Here's how the part is built. I have some questions about the finished solid (model axes, mm). Face numbers are marked on the shaded views. A direction names the side the tool comes from. Round coordinates to 2 decimals unless told otherwise and drop trailing zeros. Write each loop counter-clockwise with the first axis right and the second up, starting at its lowest first coordinate (ties: lowest second). Pieces come first, ordered by that corner, then holes. Notation, with made-up numbers: (4, 86) -> (31, 86) arc R15 cw to (31, 101) -> close; hole circle Ø10 at (83, 46). An arc over 180 degrees is marked (long way). Put each result on its own line as item: value. Start each with the question number.
1) Will these pins go through, and if not, where does the flat tip stop? P1, Ø8, axis at x = -17.5, z = 22.5, coming from the -Y side; P2, Ø8, axis at x = 16.5, z = 18, coming from the -Y side.
2) Which directions (+Z, -Z, +X, -X, +Y, -Y) give clear straight access to the entire face, cutting with the end or side of a thin tool? Please do the marked faces 1 and 2.
3) If I drill on line 1 along X through (y, z) = (-12, 22.5); line 2 along Z through (x, y) = (13.5, -4.25); line 3 along Z through (x, y) = (-27, -5.75), over which ranges is the centre line in solid material (lowest first)? Write a range as [from, to].
4) I want a section at C-C, the plane y = -9.5. List the corners of the cut face in (x, z) for me, then the cut area to 3 significant figures.
5) I want a section at B-B, the plane z = -9. List the corners of the cut face in (x, y) for me, then the cut area to 3 significant figures.
6) I want a section at A-A, the plane x = 4. List the corners of the cut face in (y, z) for me, then the cut area to 3 significant figures.
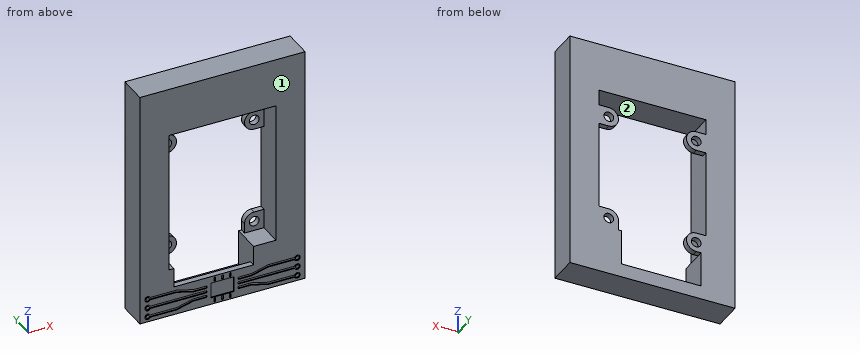
from build123d import *

# Parameters (mm, degrees)
F0_W     = 85
F0_H     = 123
F1_DEPTH = 15
F0_R     = 2.5
F2_DEPTH = 3
F3_START = 12
F0_W_2   = 41
F0_H_2   = 8
F3_DEPTH = 3
F4_R     = 0.875
F5_DEPTH = 0.5


with BuildPart() as f1:
    # F0 (on Front) → F1 (new body)
    with BuildSketch(Plane.XZ):
        with Locations((-6.7032766342, -3.7414353937)):
            Rectangle(F0_W, F0_H)
        Polygon((-34.2032766342, 24.7585646063), (-34.2032766342, 32.7585646063), (20.7967233658, 32.7585646063), (20.7967233658, 24.7585646063), (20.7967233658, 14.7585646063), (20.7967233658, -30.2414353937), (20.7967233658, -40.2414353937), (15.7967233658, -40.2414353937), (10.7967233658, -40.2414353937), (9.2967233658, -40.2414353937), (9.2967233658, -50.2414353937), (9.2967233658, -58.2414353937), (-31.7032766342, -58.2414353937), (-31.7032766342, -50.2414353937), (-31.7032766342, -40.2414353937), (-34.2032766342, -40.2414353937), (-34.2032766342, -30.2414353937), (-34.2032766342, 14.7585646063), align=None, mode=Mode.SUBTRACT)
    extrude(amount=F1_DEPTH)

    # F0 (on Front) → F2 (join)
    with BuildSketch(Plane.XZ):
        with BuildLine():
            Line((-29.2032766342, 24.7585646063), (-34.2032766342, 24.7585646063))
            Line((-34.2032766342, 24.7585646063), (-34.2032766342, 14.7585646063))
            Line((-34.2032766342, 14.7585646063), (-29.2032766342, 14.7585646063))
            ThreePointArc((-29.2032766342, 14.7585646063), (-24.2032766342, 19.7585646063), (-29.2032766342, 24.7585646063))
        make_face()
        with Locations((-29.2032766342, 19.7585646063)):
            Circle(F0_R, mode=Mode.SUBTRACT)
        with BuildLine():
            Line((20.7967233658, 14.7585646063), (20.7967233658, 24.7585646063))
            Line((20.7967233658, 24.7585646063), (15.7967233658, 24.7585646063))
            ThreePointArc((15.7967233658, 24.7585646063), (10.7967233658, 19.7585646063), (15.7967233658, 14.7585646063))
            Line((15.7967233658, 14.7585646063), (20.7967233658, 14.7585646063))
        make_face()
        with Locations((15.7967233658, 19.7585646063)):
            Circle(F0_R, mode=Mode.SUBTRACT)
        with BuildLine():
            Line((20.7967233658, -40.2414353937), (20.7967233658, -30.2414353937))
            Line((20.7967233658, -30.2414353937), (15.7967233658, -30.2414353937))
            ThreePointArc((15.7967233658, -30.2414353937), (12.2611894599, -31.7059014878), (10.7967233658, -35.2414353937))
            Line((10.7967233658, -35.2414353937), (10.7967233658, -40.2414353937))
            Line((10.7967233658, -40.2414353937), (15.7967233658, -40.2414353937))
            Line((15.7967233658, -40.2414353937), (20.7967233658, -40.2414353937))
        make_face()
        with Locations((15.7967233658, -35.2414353937)):
            Circle(F0_R, mode=Mode.SUBTRACT)
        with BuildLine():
            Line((-29.2032766342, -30.2414353937), (-34.2032766342, -30.2414353937))
            Line((-34.2032766342, -30.2414353937), (-34.2032766342, -40.2414353937))
            Line((-34.2032766342, -40.2414353937), (-31.7032766342, -40.2414353937))
            Line((-31.7032766342, -40.2414353937), (-29.2032766342, -40.2414353937))
            ThreePointArc((-29.2032766342, -40.2414353937), (-24.2032766342, -35.2414353937), (-29.2032766342, -30.2414353937))
        make_face()
        with Locations((-29.2032766342, -35.2414353937)):
            Circle(F0_R, mode=Mode.SUBTRACT)
    extrude(amount=F2_DEPTH)

    # F0 (on Front) → F3 (join)
    with BuildSketch(Plane.XZ.offset(F3_START)):
        with Locations((-11.2032766342, -54.2414353937)):
            Rectangle(F0_W_2, F0_H_2)
    extrude(amount=F3_DEPTH)

    # F4 (on face) → F5 (cut)
    with BuildSketch(Plane.XZ.offset(15)):
        with BuildLine():
            Line((-30.2032766342, -52.3664353937), (-43.8396876199, -52.3664353937))
            ThreePointArc((-43.8396876199, -52.3664353937), (-46.7032766342, -52.9914353937), (-43.8396876199, -53.6164353937))
            Line((-43.8396876199, -53.6164353937), (-30.2032766342, -53.6164353937))
            Line((-30.2032766342, -53.6164353937), (-21.7032766342, -55.8664353937))
            Line((-21.7032766342, -55.8664353937), (-15.2032766342, -55.8664353937))
            ThreePointArc((-15.2032766342, -55.8664353937), (-14.5782766342, -55.2414353937), (-15.2032766342, -54.6164353937))
            Line((-15.2032766342, -54.6164353937), (-21.7032766342, -54.6164353937))
            Line((-21.7032766342, -54.6164353937), (-30.2032766342, -52.3664353937))
        make_face()
        with Locations((-45.2032766342, -52.9914353937)):
            Circle(F4_R, mode=Mode.SUBTRACT)
        with BuildLine():
            Line((-15.2032766342, -57.1164353937), (-43.8396876199, -57.1164353937))
            ThreePointArc((-43.8396876199, -57.1164353937), (-46.7032766342, -57.7414353937), (-43.8396876199, -58.3664353937))
            Line((-43.8396876199, -58.3664353937), (-15.2032766342, -58.3664353937))
            ThreePointArc((-15.2032766342, -58.3664353937), (-14.5782766342, -57.7414353937), (-15.2032766342, -57.1164353937))
        make_face()
        with Locations((-45.2032766342, -57.7414353937)):
            Circle(F4_R, mode=Mode.SUBTRACT)
        with BuildLine():
            Line((-30.2032766342, -61.8664353937), (-43.8396876199, -61.8664353937))
            ThreePointArc((-43.8396876199, -61.8664353937), (-46.7032766342, -62.4914353937), (-43.8396876199, -63.1164353937))
            Line((-43.8396876199, -63.1164353937), (-30.2032766342, -63.1164353937))
            Line((-30.2032766342, -63.1164353937), (-21.7032766342, -60.8664353937))
            Line((-21.7032766342, -60.8664353937), (-15.2032766342, -60.8664353937))
            ThreePointArc((-15.2032766342, -60.8664353937), (-14.5782766342, -60.2414353937), (-15.2032766342, -59.6164353937))
            Line((-15.2032766342, -59.6164353937), (-21.7032766342, -59.6164353937))
            Line((-21.7032766342, -59.6164353937), (-30.2032766342, -61.8664353937))
        make_face()
        with Locations((-45.2032766342, -62.4914353937)):
            Circle(F4_R, mode=Mode.SUBTRACT)
        with BuildLine():
            Line((16.7967233658, -53.6164353937), (30.4331343515, -53.6164353937))
            ThreePointArc((30.4331343515, -53.6164353937), (33.2967233658, -52.9914353937), (30.4331343515, -52.3664353937))
            Line((30.4331343515, -52.3664353937), (16.7967233658, -52.3664353937))
            Line((16.7967233658, -52.3664353937), (8.2967233658, -54.6164353937))
            Line((8.2967233658, -54.6164353937), (1.7967233658, -54.6164353937))
            ThreePointArc((1.7967233658, -54.6164353937), (1.1717233658, -55.2414353937), (1.7967233658, -55.8664353937))
            Line((1.7967233658, -55.8664353937), (8.2967233658, -55.8664353937))
            Line((8.2967233658, -55.8664353937), (16.7967233658, -53.6164353937))
        make_face()
        with Locations((31.7967233658, -52.9914353937)):
            Circle(F4_R, mode=Mode.SUBTRACT)
        with BuildLine():
            Line((1.7967233658, -58.3664353937), (30.4331343515, -58.3664353937))
            ThreePointArc((30.4331343515, -58.3664353937), (33.2967233658, -57.7414353937), (30.4331343515, -57.1164353937))
            Line((30.4331343515, -57.1164353937), (1.7967233658, -57.1164353937))
            ThreePointArc((1.7967233658, -57.1164353937), (1.1717233658, -57.7414353937), (1.7967233658, -58.3664353937))
        make_face()
        with Locations((31.7967233658, -57.7414353937)):
            Circle(F4_R, mode=Mode.SUBTRACT)
        with BuildLine():
            Line((16.7967233658, -63.1164353937), (30.4331343515, -63.1164353937))
            ThreePointArc((30.4331343515, -63.1164353937), (33.2967233658, -62.4914353937), (30.4331343515, -61.8664353937))
            Line((30.4331343515, -61.8664353937), (16.7967233658, -61.8664353937))
            Line((16.7967233658, -61.8664353937), (8.2967233658, -59.6164353937))
            Line((8.2967233658, -59.6164353937), (1.7967233658, -59.6164353937))
            ThreePointArc((1.7967233658, -59.6164353937), (1.1717233658, -60.2414353937), (1.7967233658, -60.8664353937))
            Line((1.7967233658, -60.8664353937), (8.2967233658, -60.8664353937))
            Line((8.2967233658, -60.8664353937), (16.7967233658, -63.1164353937))
        make_face()
        with Locations((31.7967233658, -62.4914353937)):
            Circle(F4_R, mode=Mode.SUBTRACT)
        Polygon((-12.7032766342, -61.7414353937), (-6.7032766342, -61.7414353937), (-0.7032766342, -61.7414353937), (-0.7032766342, -57.7414353937), (-0.7032766342, -53.7414353937), (-6.7032766342, -53.7414353937), (-12.7032766342, -53.7414353937), (-12.7032766342, -57.7414353937), align=None)
        with BuildLine():
            Line((-6.2032766342, -52.7414353937), (-6.2032766342, -51.4914353937))
            ThreePointArc((-6.2032766342, -51.4914353937), (-6.7032766342, -50.9914353937), (-7.2032766342, -51.4914353937))
            Line((-7.2032766342, -51.4914353937), (-7.2032766342, -52.7414353937))
            ThreePointArc((-7.2032766342, -52.7414353937), (-6.7032766342, -53.2414353937), (-6.2032766342, -52.7414353937))
        make_face()
        with BuildLine():
            Line((-2.2032766342, -52.7414353937), (-2.2032766342, -51.4914353937))
            ThreePointArc((-2.2032766342, -51.4914353937), (-2.7032766342, -50.9914353937), (-3.2032766342, -51.4914353937))
            Line((-3.2032766342, -51.4914353937), (-3.2032766342, -52.7414353937))
            ThreePointArc((-3.2032766342, -52.7414353937), (-2.7032766342, -53.2414353937), (-2.2032766342, -52.7414353937))
        make_face()
        with BuildLine():
            ThreePointArc((-11.2032766342, -52.7414353937), (-10.7032766342, -53.2414353937), (-10.2032766342, -52.7414353937))
            Line((-10.2032766342, -52.7414353937), (-10.2032766342, -51.4914353937))
            ThreePointArc((-10.2032766342, -51.4914353937), (-10.7032766342, -50.9914353937), (-11.2032766342, -51.4914353937))
            Line((-11.2032766342, -51.4914353937), (-11.2032766342, -52.7414353937))
        make_face()
        with BuildLine():
            Line((-11.2032766342, -62.7414353937), (-11.2032766342, -63.9914353937))
            ThreePointArc((-11.2032766342, -63.9914353937), (-10.7032766342, -64.4914353937), (-10.2032766342, -63.9914353937))
            Line((-10.2032766342, -63.9914353937), (-10.2032766342, -62.7414353937))
            ThreePointArc((-10.2032766342, -62.7414353937), (-10.7032766342, -62.2414353937), (-11.2032766342, -62.7414353937))
        make_face()
        with BuildLine():
            Line((-3.2032766342, -62.7414353937), (-3.2032766342, -63.9914353937))
            ThreePointArc((-3.2032766342, -63.9914353937), (-2.7032766342, -64.4914353937), (-2.2032766342, -63.9914353937))
            Line((-2.2032766342, -63.9914353937), (-2.2032766342, -62.7414353937))
            ThreePointArc((-2.2032766342, -62.7414353937), (-2.7032766342, -62.2414353937), (-3.2032766342, -62.7414353937))
        make_face()
        with BuildLine():
            ThreePointArc((-6.2032766342, -62.7414353937), (-6.7032766342, -62.2414353937), (-7.2032766342, -62.7414353937))
            Line((-7.2032766342, -62.7414353937), (-7.2032766342, -63.9914353937))
            ThreePointArc((-7.2032766342, -63.9914353937), (-6.7032766342, -64.4914353937), (-6.2032766342, -63.9914353937))
            Line((-6.2032766342, -63.9914353937), (-6.2032766342, -62.7414353937))
        make_face()
    extrude(amount=-F5_DEPTH, mode=Mode.SUBTRACT)


solid = f1.part
Findings:
1. P1: passes through
1. P2: stops at y = -3
2. face 1: +Z, -Z, +X, -X, -Y
2. face 2: +Y, -Y
3. line 1: x = [-49.2, -34.2], [20.8, 35.8]
3. line 2: z = [-65.24, -40.24], [32.76, 57.76]
3. line 3: z = [-65.24, -58.24], [32.76, 57.76]
4. outline: (-49.2, -65.24) -> (35.8, -65.24) -> (35.8, 57.76) -> (-49.2, 57.76) -> close; hole (-34.2, -40.24) -> (-31.7, -40.24) -> (-31.7, -58.24) -> (9.3, -58.24) -> (9.3, -40.24) -> (20.8, -40.24) -> (20.8, 32.76) -> (-34.2, 32.76) -> close
4. area: 5,700 mm2
5. outline: (-49.2, -15) -> (-34.2, -15) -> (-34.2, 0) -> (-49.2, 0) -> close; (20.8, -15) -> (35.8, -15) -> (35.8, 0) -> (20.8, 0) -> close
5. area: 450 mm2
6. outline: (-15, -65.24) -> (0, -65.24) -> (0, -58.24) -> (-12, -58.24) -> (-12, -50.24) -> (-15, -50.24) -> (-15, -54.62) -> (-14.5, -54.62) -> (-14.5, -55.87) -> (-15, -55.87) -> (-15, -57.12) -> (-14.5, -57.12) -> (-14.5, -58.37) -> (-15, -58.37) -> (-15, -59.62) -> (-14.5, -59.62) -> (-14.5, -60.87) -> (-15, -60.87) -> close; (-15, 32.76) -> (0, 32.76) -> (0, 57.76) -> (-15, 57.76) -> close
6. area: 502 mm2
